Part model, mm, in its own coordinate system. Give positions to 0.01 mm unless a question says otherwise; leave off trailing zeros. Write each loop counter-clockwise with the first axis right and the second up, starting at its lowest first coordinate (ties: lowest second). Pieces come first, ordered by that corner, then holes. Notation, with made-up numbers: M 24,88 L 80,88 A36 cw 80,122 Z; hole C 65,7 d9. An arc over 180 degrees is marked long. Answer as CSV lines item,"result". Start each with the question number.
Item 1: Band-saw the part on A-A, the plane x = 3.05. List the corners of the cut face in (y, z) (3 decimals), then the cut area to 3 significant figures.
Item 2: Band-saw the part on D-D, the plane x = 2. List the corners of the cut face in (y, z) (3 decimals).
Item 3: Pin check, flat tips, straight feed: pin 1 (2 mm diameter, centred on x = 4, z = 3.5, fed in from +Y); pin 2 (2 mm diameter, centred on y = 8.5, z = 0, fed in from -X); pin 3 (1.3 mm diameter, centred on x = 3, y = 5.5, fed in from +Z). Stop position of each tip, or through.
Item 4: Band-saw the part on C-C, the plane y = 8.25. List the corners of the cut face in (x, z).
Item 5: Wall check: L1, parallel to Z at x = 3.5, y = 5.5; L2, parallel to Z at x = 2, y = 6.25; L3, parallel to Y at x = 4.35, z = -4.5. Give the ranges that are in metal, low to high. Write a range as from..to.
Item 6: Band-saw the part on B-B, the plane z = -2. List the corners of the cut face in (x, y), then the cut area to 3 significant figures.
from build123d import *

# Parameters (mm, degrees)
HOOK_LEVER_DEPTH      = 1.8
HOOK_LEVER_DEPTH_BACK = 1.8
CUT_DEPTH             = 14.210060999


with BuildPart() as part:
    # Эскиз1 → Hook_Lever (new, two sides: drawn at the far end of the back side and taken through both)
    with BuildSketch(Plane(origin=(2.85, 0, 0), x_dir=(0, 0, -1), z_dir=(1, 0, 0)).offset(-HOOK_LEVER_DEPTH_BACK)):
        with BuildLine():
            Line((5.55, 4.85), (5.55, 6.042820323))
            ThreePointArc((5.55, 6.042820323), (5.450943953, 6.341557576), (5.193024215, 6.521927904))
            Line((5.193024215, 6.521927904), (-8.144994918, 10.50362176))
            ThreePointArc((-8.144994918, 10.50362176), (-8.427699037, 10.639328236), (-8.654473244, 10.855918461))
            ThreePointArc((-8.654473244, 10.855918461), (-9.625040353, 11.23456126), (-10.40562376, 10.544589936))
            Line((-10.40562376, 10.544589936), (-10.548967324, 10.588778426))
            ThreePointArc((-10.548967324, 10.588778426), (-9.651296406, 11.382245449), (-8.535144231, 10.94680623))
            ThreePointArc((-8.535144231, 10.94680623), (-8.342386155, 10.762704538), (-8.102087654, 10.647354034))
            Line((-8.102087654, 10.647354034), (5.235931479, 6.665660178))
            ThreePointArc((5.235931479, 6.665660178), (5.571227139, 6.431178752), (5.7, 6.042820323))
            Line((5.7, 6.042820323), (5.7, 4.85))
            Line((5.7, 4.85), (5.55, 4.85))
        make_face()
    extrude(amount=HOOK_LEVER_DEPTH + HOOK_LEVER_DEPTH_BACK)

    # Эскиз2 → Cut (cut, through all)
    with BuildSketch(Plane(origin=(0, 4.95, 0), x_dir=(1, 0, 0), z_dir=(0, 1, 0))):
        Polygon((1.05, 5.8), (1.35, -10.548967324), (1.05, -10.548967324), align=None)
        Polygon((4.65, 5.8), (4.65, -10.548967324), (4.35, -10.548967324), align=None)
        with BuildLine():
            Line((2.35, 5.8), (3.35, 5.8))
            Line((3.35, 5.8), (3.20551955, -1.905624011))
            ThreePointArc((3.20551955, -1.905624011), (3.115706509, -2.11411119), (2.90557227, -2.2))
            Line((2.90557227, -2.2), (2.79442773, -2.2))
            ThreePointArc((2.79442773, -2.2), (2.584293491, -2.11411119), (2.49448045, -1.905624011))
            Line((2.49448045, -1.905624011), (2.35, 5.8))
        make_face()
    extrude(amount=CUT_DEPTH, mode=Mode.SUBTRACT)


solid = part.part
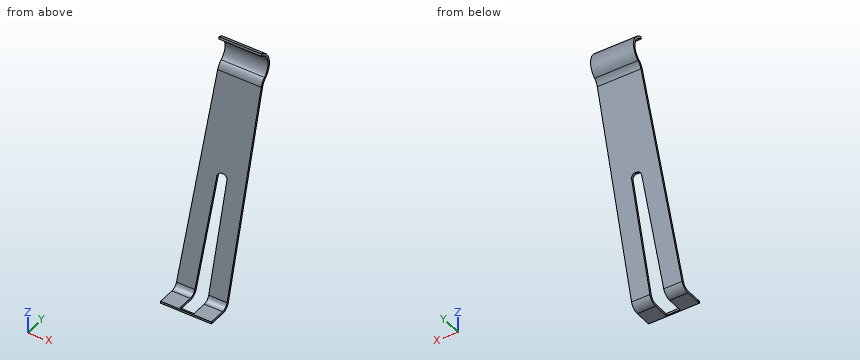
Output:
1,outline,"M 4.85,-5.7 L 4.95,-5.7 L 4.95,-5.55 L 4.85,-5.55 Z; M 8.718,2.163 L 8.874,2.163 L 10.647,8.102 A0.85 cw 10.947,8.535 A1.15 ccw 10.589,10.549 L 10.545,10.406 A1 cw 10.856,8.654 A1 ccw 10.504,8.145 Z"
1,area,"1.39 mm²"
2,outline,"M 4.85,-5.7 L 6.043,-5.7 A0.65 ccw 6.666,-5.236 L 10.647,8.102 A0.85 cw 10.947,8.535 A1.15 ccw 10.589,10.549 L 10.545,10.406 A1 cw 10.856,8.654 A1 ccw 10.504,8.145 L 6.522,-5.193 A0.5 cw 6.043,-5.55 L 4.85,-5.55 Z"
3,pin 1,"y = 9.57"
3,pin 2,"x = 1.14"
3,pin 3,"z = -5.55"
4,outline,"M 1.16,0.07 L 2.46,0.07 L 2.47,0.6 L 1.17,0.6 Z; M 3.23,0.6 L 3.24,0.07 L 4.54,0.07 L 4.53,0.6 Z"
5,L1,"-5.7..-5.55"
5,L2,"-5.67..-5.51"
5,L3,"6.73..6.89"
6,outline,"M 1.12,7.48 L 2.42,7.48 L 2.42,7.63 L 1.12,7.63 Z; M 3.28,7.48 L 4.58,7.48 L 4.58,7.63 L 3.28,7.63 Z"
6,area,"0.407 mm²"
